The model under review builds one solid part; all positions refer to its coordinate system, in mm. Face numbers are marked on the shaded views. Round coordinates to 2 decimals unless told otherwise and drop trailing zeros. Write each loop counter-clockwise with the first axis right and the second up, starting at its lowest first coordinate (ties: lowest second). Pieces come first, ordered by that corner, then holes. Notation, with made-up numbers: (-38, 71) -> (-5, 71) arc R20 ccw to (-5, 79) -> close; hole circle Ø10 at (29, 56). An arc over 180 degrees is marked (long way). Return JSON: item names as keys, results as strings. Group by question number.
1. For line 1 along Y through (x, z) = (13.5, -8); line 2 along X through (y, z) = (6, -12.5); line 3 along Z through (x, y) = (-6, 2), list the stretches that pass through material, from the lowest coordinate up. Write a range as from..to.
2. Clearance check with flat-ended pins moving along their axes: P1, Ø2, axis at y = 8.5, z = 4.5, coming from the -X side; P2, Ø17.5, axis at x = -8.5, z = -3.5, coming from the -Y side; P3, Ø1.5, axis at x = 6.5, y = 8.5, coming from the +Z side; P4, Ø5, axis at x = 15, y = 1.5, coming from the -Z side. State where each tip first meets the part, or that it passes through.
3. Take a section at C-C, the plane y = 2. Write out the cut boundary in (x, z), then the cut area to 3 significant figures.
4. Mouldability with a two-part tool opening along Z and no side actions: class the marked faces 1, 2 and 3 as pulls with the +Z half, pulls with the -Z half, needs draft (parallel to the pull), parting line crosses it, or undercut.
5. Take a section at D-D, the plane y = 7.5. Write out the cut boundary in (x, z) (1 decimal).
Autodesk Inventor part; units mm, degrees
ref_plane "YZ Plane" through (0, 0, 0) normal (1, 0, 0) x (0, 1, 0)
ref_plane "XZ Plane" through (0, 0, 0) normal (0, 1, 0) x (-1, 0, 0)
ref_plane "XY Plane" through (0, 0, 0) normal (0, 0, 1) x (1, 0, 0)
sketch "Skizze1" plane through (0, 0, 0) normal (0, 0, 1) x (1, 0, 0)
  line L0 (10, 12) -> (20, 12)
  line L1 (20, 12) -> (19.5, 0)
  line L2 (19.5, 0) -> (17.5, 0)
  line L3 (17.5, 0) -> (17.5, 10)
  line L4 (17.5, 10) -> (10, 10)
  line L5 (10, 10) -> (10, 12)
  line L6 (0, 0) -> (0, 8.6013)
  line L7 (18.5, 0) -> (18.5, 1.5)
  line L8 (18.5, 1.5) -> (17.5, 1.5)
  dimension "d0" = 35
  dimension "d1" = 10
  dimension "d2" = 20
  dimension "d4" = 2
  dimension "d9" = 10
  dimension "d10" = 2
  dimension "d15" = 1
  dimension "d16" = 1.5
revolve "Umdrehung1" add sketch "Skizze1" angle 360 about axis through (0, 0, 0) along (0, 1, 0)
chamfer "Fasen1" distance 2 angle 45 1 edges at (-10, 12, 0)
thread "Gewinde1"
fillet "Rundung1" radius 3 1 edges at (-20, 12, 0)
fillet "Rundung2" radius 1 1 edges at (-19.5, 0, 0)
properties part number "Deckel"
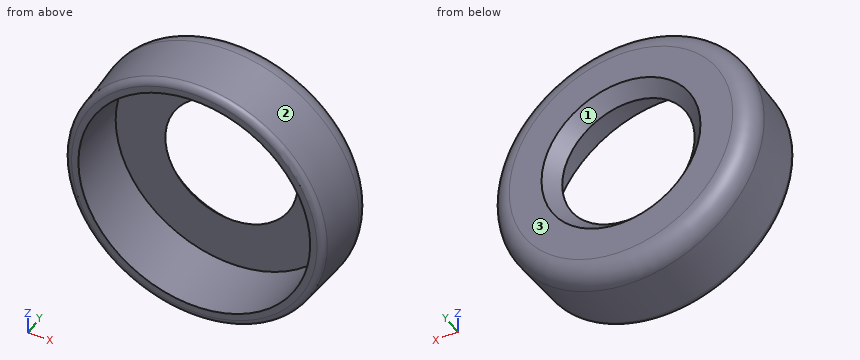
Output:
{
 "1": {"line 1": "y = 10..12", "line 2": "x = -15.29..-12.25, 12.25..15.29", "line 3": "z = -18.64..-16.44, 16.44..18.64"},
 "2": {"P1": "stops at x = -19.55", "P2": "stops at y = 0", "P3": "stops at z = 19.01", "P4": "stops at z = -15.05"},
 "3": {"outline": "circle Ø39.17 at (0, 0); hole circle Ø35 at (0, 0)", "area": "243 mm^2"},
 "4": {"face 1": "undercut", "face 2": "parting line crosses it", "face 3": "needs draft"},
 "5": {"outline": "circle Ø39.6 at (0, 0); hole circle Ø35 at (0, 0)"}
}
